Could you check a few things on this model? Use its own coordinates, in mm. Face numbers are marked on the shaded views. A direction names the side the tool comes from. Give positions to 0.01 mm unless a question says otherwise; leave off trailing zeros. Loops run counter-clockwise (first coordinate to the right, second up) from the corner with the lowest first, then second, coordinate; pieces in that order, holes last. Notation, with made-up numbers: (40.25, -6.75) -> (73.25, -6.75) arc R16 ccw to (73.25, 6.25) -> close; hole circle Ø7 at (28.5, -19.75). An arc over 180 degrees is marked (long way). Write each question's results on one line, items separated by ' | '. Start each with the question number.
Q1. If I drill on line 1 along Y through (x, z) = (-24.3, 5); line 2 along X through (y, z) = (5.5, -3.5); line 3 along Y through (x, z) = (-21.5, -3), over which ranges is the centre line in solid material (lowest first)?
Q2. We'd pull the mould along X, two halves only. Please class the marked faces 1, 2 and 3: released by +X, released by -X, zero draft, split by the parting line, or undercut.
Q3. Will these pins go through, and if not, where does the flat tip stop? P1, Ø2.5, axis at y = 6, z = -1.5, coming from the +X side; P2, Ø1.8, axis at x = -20.5, z = -0.5, coming from the +Y side; P3, Ø6, axis at x = -12.5, z = 4.5, coming from the -Y side.
Q4. If we section it at C-C, the plane z = 5: List the corners of the cut face in (x, y) for me.
Q5. If we section it at A-A, the plane y = 4.25: Give the number of separate pieces and of enclosed holes in the cut face, plus the area to 3 significant figures.
Q6. Which directions (+Z, -Z, +X, -X, +Y, -Y) give clear straight access to the entire face, cutting with the end or side of a thin tool? Please do the marked faces 4, 5 and 6.
Q7. If we section it at B-B, the plane x = -18.5: List the corners of the cut face in (y, z) for me.
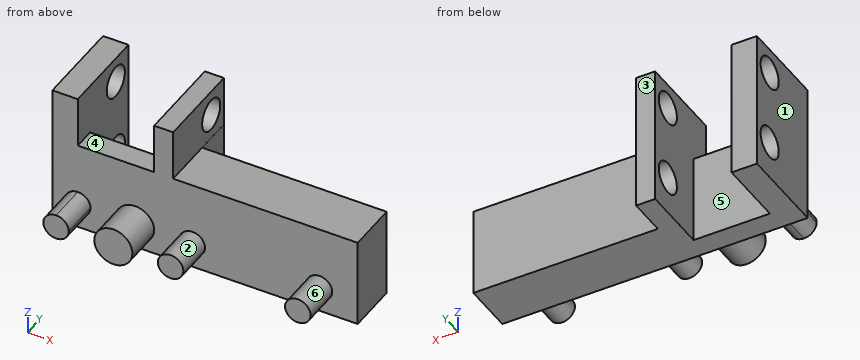
from build123d import *

# Parameters (mm, degrees)
BOSS_EXTRUDE1_DEPTH = 3
SKETCH3_W           = 24
SKETCH3_H           = 4
BOSS_EXTRUDE2_DEPTH = 4
SKETCH6_W           = 24
SKETCH6_H           = 4
BOSS_EXTRUDE4_DEPTH = 3
CUT_EXTRUDE1_DEPTH  = 2.3
SKETCH9_W           = 2
SKETCH9_H           = 7
SKETCH9_W_2         = 1.5
BOSS_EXTRUDE5_DEPTH = 3
SKETCH11_W          = 2
SKETCH11_H          = 7
SKETCH11_W_2        = 1.497470588
BOSS_EXTRUDE6_DEPTH = 4
SKETCH10_R          = 1.25
CUT_EXTRUDE2_DEPTH  = 10.5


with BuildPart() as part:
    # Sketch1 → Boss-Extrude1 (new body)
    with BuildSketch(Plane(origin=(0, 0, 0), x_dir=(1, 0, 0), z_dir=(0, 1, 0))):
        with BuildLine():
            ThreePointArc((-17, 2), (-18.5, 3.5), (-20, 2))
            Line((-20, 2), (-17, 2))
        make_face()
        with BuildLine():
            Line((-17, 2), (-20, 2))
            ThreePointArc((-20, 2), (-18.5, 0.5), (-17, 2))
        make_face()
        with BuildLine():
            Line((-23, 3), (-23, 2))
            Line((-23, 2), (-23, 1))
            ThreePointArc((-23, 1), (-22.292893219, 1.292893219), (-22, 2))
            ThreePointArc((-22, 2), (-22.292893219, 2.707106781), (-23, 3))
        make_face()
        with BuildLine():
            Line((-23, 1), (-23, 2))
            Line((-23, 2), (-24, 2))
            ThreePointArc((-24, 2), (-23.707106781, 1.292893219), (-23, 1))
        make_face()
        with BuildLine():
            Line((-24, 2), (-23, 2))
            Line((-23, 2), (-23, 3))
            ThreePointArc((-23, 3), (-23.707106781, 2.707106781), (-24, 2))
        make_face()
        with BuildLine():
            ThreePointArc((-13, 2), (-14, 3), (-15, 2))
            Line((-15, 2), (-13, 2))
        make_face()
        with BuildLine():
            Line((-13, 2), (-15, 2))
            ThreePointArc((-15, 2), (-14, 1), (-13, 2))
        make_face()
        with BuildLine():
            ThreePointArc((-3, 2), (-4, 3), (-5, 2))
            Line((-5, 2), (-3, 2))
        make_face()
        with BuildLine():
            Line((-3, 2), (-5, 2))
            ThreePointArc((-5, 2), (-4, 1), (-3, 2))
        make_face()
    extrude(amount=-BOSS_EXTRUDE1_DEPTH)

    # Sketch3 → Boss-Extrude2 (add)
    with BuildSketch(Plane(origin=(0, 0, 0), x_dir=(1, 0, 0), z_dir=(0, 1, 0))):
        with Locations((-13, 2)):
            Rectangle(SKETCH3_W, SKETCH3_H)
    extrude(amount=BOSS_EXTRUDE2_DEPTH)

    # Sketch6 → Boss-Extrude4 (add)
    with BuildSketch(Plane.XY):
        with Locations((-13, 2)):
            Rectangle(SKETCH6_W, SKETCH6_H)
    extrude(amount=BOSS_EXTRUDE4_DEPTH)

    # Sketch7 → Cut-Extrude1 (cut)
    with BuildSketch(Plane(origin=(0, 4, 0), x_dir=(1, 0, 0), z_dir=(0, 1, 0))):
        Polygon((-23, 0.5), (-23, -3), (-17, -3), (-17, 4), (-23, 4), align=None)
    extrude(amount=-CUT_EXTRUDE1_DEPTH, mode=Mode.SUBTRACT)

    # Sketch9 → Boss-Extrude5 (add)
    with BuildSketch(Plane(origin=(0, 4, 0), x_dir=(1, 0, 0), z_dir=(0, 1, 0))):
        with Locations((-24, 0.5)):
            Rectangle(SKETCH9_W, SKETCH9_H)
        with Locations((-16.25, 0.5)):
            Rectangle(SKETCH9_W_2, SKETCH9_H)
    extrude(amount=BOSS_EXTRUDE5_DEPTH)

    # Sketch11 → Boss-Extrude6 (add)
    with BuildSketch(Plane.XY.offset(3)):
        with Locations((-24, 3.5)):
            Rectangle(SKETCH11_W, SKETCH11_H)
        with Locations((-16.251264706, 3.5)):
            Rectangle(SKETCH11_W_2, SKETCH11_H)
    extrude(amount=BOSS_EXTRUDE6_DEPTH)

    # Sketch10 → Cut-Extrude2 (cut, through all)
    with BuildSketch(Plane(origin=(-15.5, 0, 0), x_dir=(0, 0, -1), z_dir=(1, 0, 0))):
        with Locations((1, 5.25)):
            Circle(SKETCH10_R)
        with Locations((-5, 5.25)):
            Circle(SKETCH10_R)
    extrude(amount=-CUT_EXTRUDE2_DEPTH, mode=Mode.SUBTRACT)


solid = part.part
Final values:
1) line 1: y = 0 to 4, 6.5 to 7 | line 2: x = -25 to -23, -17 to -15.5 | line 3: y = 0 to 1.7
2) face 1: released by -X | face 2: undercut | face 3: zero draft
3) P1: stops at x = -15.5 | P2: stops at y = 1.7 | P3: stops at y = 0
4) outline: (-25, 0) -> (-23, 0) -> (-23, 4) -> (-25, 4) -> close; (-25, 6.5) -> (-23, 6.5) -> (-23, 7) -> (-25, 7) -> close; (-17, 0) -> (-15.5, 0) -> (-15.5, 4) -> (-17, 4) -> close; (-17, 6.5) -> (-15.5, 6.5) -> (-15.5, 7) -> (-17, 7) -> close
5) separate pieces: 6 | enclosed holes: 0 | area: 28.0 mm²
6) face 4: +Z, +Y, -Y | face 5: +Z, -Z, +Y | face 6: -Y
7) outline: (-3, -3.5) -> (0, -3.5) -> (0, -4) -> (1.7, -4) -> (1.7, 3) -> (0, 3) -> (0, -0.5) -> (-3, -0.5) -> close
